CAD build for the part. Positions are in the model's coordinates, mm. A direction names the side the tool comes from. Give positions to 0.01 mm unless a question says otherwise; leave off trailing zeros. Loops run counter-clockwise (first coordinate to the right, second up) from the corner with the lowest first, then second, coordinate; pieces in that order, holes last.
Item 1: Probe probe 1 along X at (y, z) = (49, 3.5); probe 2 along Y at (x, z) = (84, 13.5); probe 3 along Z at (x, y) = (16, 18.5). List the from-to ranges inside material, lowest first.
Item 2: Saw through at B-B on x = 87. Give the cut face in (y, z).
Item 3: Saw through at D-D on y = 25.5. Give the cut face in (x, z), plus the area to 3 significant figures.
Item 4: Saw through at A-A on y = 44.5. Give the cut face in (x, z), plus the area to 3 significant figures.
Item 5: Which spindle directions (+Z, -Z, +X, -X, +Y, -Y) get a long thin tool onto all of the face, cutting with end or side? Do faces 1 (the flat face through (24, 28, -8)), 2 (the flat face through (81, 42, 8)), 3 (the flat face through (72, 41, 10)), 4 (the flat face through (12, 14, -21)). Say none if no direction does.
Item 6: Saw through at C-C on z = -6.5. Give the cut face in (x, y).
Item 7: Drop flat-ended pins along their axis: P1, Ø4, axis at x = 114, z = 0.5, coming from the +Y side; P2, Ø15.5, axis at x = 38, z = -18.5, coming from the +Y side; P3, Ø5, axis at y = 42, z = 12, coming from the -X side; P4, Ø17.5, axis at x = 73, y = 37.5, coming from the -Z side. Give the stop position or say it passes through.
from build123d import *

# Parameters (mm, degrees)
SKETCH1_W           = 31.35
SKETCH1_H           = 28
BOSS_EXTRUDE1_DEPTH = 12
SKETCH2_W           = 10
SKETCH2_H           = 28
BOSS_EXTRUDE2_DEPTH = 120
SKETCH3_W           = 60
SKETCH3_H           = 25
BOSS_EXTRUDE3_DEPTH = 10
SKETCH4_W           = 42
SKETCH4_H           = 22
CUT_EXTRUDE1_DEPTH  = 146.656522339
BOSS_EXTRUDE4_DEPTH = 17
CHAMFER1_SIZE       = 10
SKETCH6_W           = 10
SKETCH6_H           = 22
CUT_EXTRUDE2_DEPTH  = 9
CHAMFER2_SIZE       = 10


with BuildPart() as part:
    # Sketch1 → Boss-Extrude1 (new body)
    with BuildSketch(Plane(origin=(0, 0, 0), x_dir=(0, 0, -1), z_dir=(1, 0, 0))):
        with Locations((15.675, 14)):
            Rectangle(SKETCH1_W, SKETCH1_H)
    extrude(amount=BOSS_EXTRUDE1_DEPTH)

    # Sketch2 → Boss-Extrude2 (add)
    with BuildSketch(Plane(origin=(12, 0, 0), x_dir=(0, 0, -1), z_dir=(1, 0, 0))):
        with Locations((5, 14)):
            Rectangle(SKETCH2_W, SKETCH2_H)
    extrude(amount=BOSS_EXTRUDE2_DEPTH)

    # Sketch3 → Boss-Extrude3 (add)
    with BuildSketch(Plane.XY):
        with Locations((102, 40.5)):
            Rectangle(SKETCH3_W, SKETCH3_H)
    extrude(amount=-BOSS_EXTRUDE3_DEPTH)

    # Sketch4 → Cut-Extrude1 (cut, through all)
    with BuildSketch(Plane.XY):
        with Locations((102, 42)):
            Rectangle(SKETCH4_W, SKETCH4_H)
    extrude(amount=-CUT_EXTRUDE1_DEPTH, mode=Mode.SUBTRACT)

    # Sketch5 → Boss-Extrude4 (add)
    with BuildSketch(Plane.XY):
        Polygon((81, 31), (81, 53), (72, 53), (72, 28), (72, 21), (132, 21), (132, 53), (123, 53), (123, 31), align=None)
    extrude(amount=BOSS_EXTRUDE4_DEPTH)

    # Chamfer1
    chamfer1_edges = [part.edges().sort_by_distance(p)[0] for p in [
        (72, 24.5, 0),
        (102, 21, 0),
    ]]
    chamfer(chamfer1_edges, length=CHAMFER1_SIZE)

    # Sketch6 → Cut-Extrude2 (cut)
    with BuildSketch(Plane.ZY.offset(-72)):
        with Locations((-5, 42)):
            Rectangle(SKETCH6_W, SKETCH6_H)
    extrude(amount=-CUT_EXTRUDE2_DEPTH, mode=Mode.SUBTRACT)

    # Chamfer2
    chamfer2_edges = [part.edges().sort_by_distance(p)[0] for p in [
        (72, 28, 0),
    ]]
    chamfer(chamfer2_edges, length=CHAMFER2_SIZE - 0.0001)  # a hair under: the kernel refuses the full size


solid = part.part
Results below:
1. probe 1: x = 72 to 81, 123 to 132
1. probe 2: y = 21 to 31
1. probe 3: z = -10 to 0
2. outline: (0, -10) - (31, -10) - (31, 17) - (21, 17) - (21, 10) - (11, 0) - (0, 0) - close
3. outline: (0, -31.35) - (12, -31.35) - (12, -10) - (132, -10) - (132, 17) - (72, 17) - (72, 10) - (62, 0) - (0, 0) - close
3. area: 2,650 mm2
4. outline: (72, 0) - (81, 0) - (81, 17) - (72, 17) - close; (123, -10) - (132, -10) - (132, 17) - (123, 17) - close
4. area: 396 mm2
5. face 1: +Z, -Z, -X, +Y
5. face 2: +Z, -Z, +Y
5. face 3: +Z, -X, +Y
5. face 4: -Z, +X, +Y, -Y
6. outline: (0, 0) - (132, 0) - (132, 53) - (123, 53) - (123, 31) - (65, 31) - (62, 28) - (0, 28) - close
7. P1: stops at y = 31
7. P2: passes through
7. P3: stops at x = 72
7. P4: stops at z = -10
